Verification items for this drawing (mm, ordinates from the low corner). A direction names the side the tool comes from. Give positions to 0.01 mm unless a question says otherwise; leave off trailing zeros. Write each loop counter-clockwise with the first axis right and the second up, starting at its lowest first coordinate (ties: lowest second). Pieces come first, ordered by that corner, then holes. Notation, with made-up numbers: (64.5, 42.5) -> (101.5, 42.5) arc R32 ccw to (101.5, 68.5) -> close; hole circle Ø8 at (55, 43). An arc over 180 degrees is marked (long way). Answer as a JSON object with one key per item and string values.
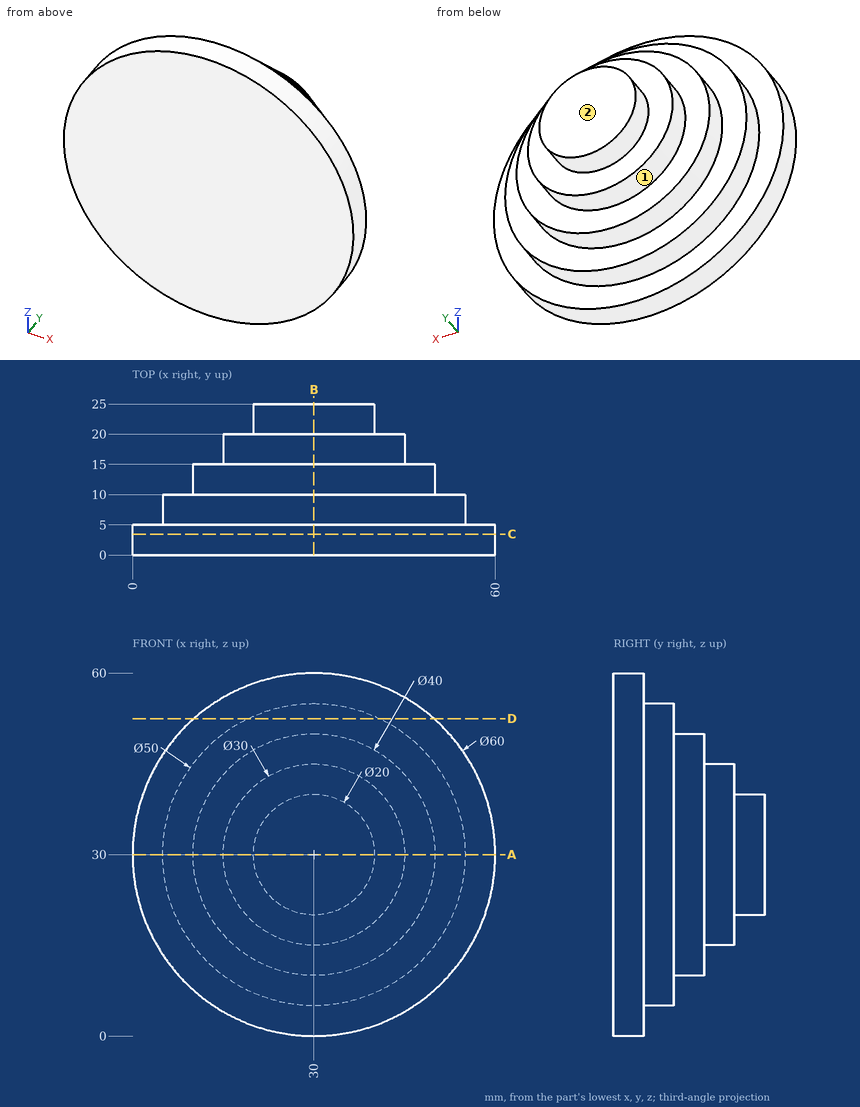
1. Sectioned sample at B-B, the plane x = 30. Enter the section's corners in (y, z), plus the area to 3 significant figures.
Determined:
{"outline": "(0, 0) -> (5, 0) -> (5, 5) -> (10, 5) -> (10, 10) -> (15, 10) -> (15, 15) -> (20, 15) -> (20, 20) -> (25, 20) -> (25, 40) -> (20, 40) -> (20, 45) -> (15, 45) -> (15, 50) -> (10, 50) -> (10, 55) -> (5, 55) -> (5, 60) -> (0, 60) -> close", "area": "1,000 mm^2"}
2. Sectioned sample at D-D, the plane z = 52.5. Enter the section's corners in (x, y), plus the area to 3 significant figures.
Determined:
{"outline": "(10.16, 0) -> (49.84, 0) -> (49.84, 5) -> (40.9, 5) -> (40.9, 10) -> (19.1, 10) -> (19.1, 5) -> (10.16, 5) -> close", "area": "307 mm^2"}
3. Go/stop test with flat-tipped pins: P1, Ø3, axis at x = 10, y = 5.5, coming from the +Z side; P2, Ø4, axis at y = 6, z = 16, coming from the -X side; P3, Ø10, axis at y = 4.5, z = 36.5, coming from the +X side. Record where each tip stops, or that it passes through.
Determined:
{"P1": "z = 53.55", "P2": "x = 2.62", "P3": "x = 59.96"}
4. Access from +Z, -Z, +X, -X, +Y, -Y to the whole of each face (thin tool, end or side, straight path). Record for the marked faces 1 and 2.
Determined:
{"face 1": "+Y", "face 2": "+Z, -Z, +X, -X, +Y"}
5. Sectioned sample at A-A, the plane z = 30. Enter the section's corners in (x, y), plus the area to 3 significant figures.
Determined:
{"outline": "(0, 0) -> (60, 0) -> (60, 5) -> (55, 5) -> (55, 10) -> (50, 10) -> (50, 15) -> (45, 15) -> (45, 20) -> (40, 20) -> (40, 25) -> (20, 25) -> (20, 20) -> (15, 20) -> (15, 15) -> (10, 15) -> (10, 10) -> (5, 10) -> (5, 5) -> (0, 5) -> close", "area": "1,000 mm^2"}
6. Scan lines: L1, parallel to Y at x = 48, z = 31.5; L2, parallel to Y at x = 57, z = 30; L3, parallel to Z at x = 26.5, y = 16.25. Record each from-to range of solid material in increasing order. Write a range as [from, to].
Determined:
{"L1": "[0, 15]", "L2": "[0, 5]", "L3": "[15.41, 44.59]"}
7. Sectioned sample at C-C, the plane y = 3.5. Enter the section's corners in (x, z), plus the area to 3 significant figures.
Determined:
{"outline": "circle Ø60 at (30, 30)", "area": "2,830 mm^2"}
